```python
from build123d import *

# Parameters (mm, degrees)
SKETCH_1_W          = 29
SKETCH_1_H          = 40
EXTRUDE_1_DEPTH     = 2
SKETCH_2_W          = 2
SKETCH_2_H          = 5
EXTRUDE_2_DEPTH     = 3.5
SKETCH_3_W          = 8.3
SKETCH_3_H          = 3.2
CUT_EXTRUDE_1_DEPTH = 50.71166865
SKETCH_4_R          = 1.9
CUT_EXTRUDE_2_DEPTH = 50.71166865
SKETCH_5_W          = 10.7
SKETCH_5_H          = 5.6
SKETCH_5_W_2        = 8.3
SKETCH_5_H_2        = 3.2
EXTRUDE_3_DEPTH     = 2
SKETCH_6_R          = 3.1
SKETCH_6_R_2        = 1.9
EXTRUDE_4_DEPTH     = 1
EXTRUDE_5_DEPTH     = 1.25
FILLET_1_R          = 0.5
FILLET_2_R          = 0.5
CHAMFER_1_SIZE      = 0.2
CHAMFER_2_SIZE      = 0.5
FILLET_3_R          = 1
FILLET_4_R          = 1
SKETCH_9_W          = 29
SKETCH_9_H          = 19
CUT_EXTRUDE_3_DEPTH = 0.6
FILLET_5_R          = 1


with BuildPart() as part:
    # 草图1 → 凸台-拉伸1 (new body)
    with BuildSketch(Plane.XY):
        with Locations((14.5, 20)):
            Rectangle(SKETCH_1_W, SKETCH_1_H)
    extrude(amount=EXTRUDE_1_DEPTH)

    # 草图2 → 凸台-拉伸2 (add)
    with BuildSketch(Plane(origin=(0, 0, 0), x_dir=(-1, 0, 0), z_dir=(0, 0, -1))):
        with Locations((-1, 34.8)):
            Rectangle(SKETCH_2_W, SKETCH_2_H)
        with Locations((-28, 34.8)):
            Rectangle(SKETCH_2_W, SKETCH_2_H)
        with Locations((-1, 5.2)):
            Rectangle(SKETCH_2_W, SKETCH_2_H)
        with Locations((-28, 5.2)):
            Rectangle(SKETCH_2_W, SKETCH_2_H)
    extrude(amount=EXTRUDE_2_DEPTH)

    # 草图3 → 切除-拉伸1 (cut, through all)
    with BuildSketch(Plane.XY.offset(2)):
        with Locations((14.5, 32.9)):
            Rectangle(SKETCH_3_W, SKETCH_3_H)
    extrude(amount=-CUT_EXTRUDE_1_DEPTH, mode=Mode.SUBTRACT)

    # 草图4 → 切除-拉伸2 (cut, through all)
    with BuildSketch(Plane.XY.offset(2)):
        with Locations((14.5, 5.2)):
            Circle(SKETCH_4_R)
        with Locations((6.2, 5.2)):
            Circle(SKETCH_4_R)
        with Locations((22.8, 5.2)):
            Circle(SKETCH_4_R)
    extrude(amount=-CUT_EXTRUDE_2_DEPTH, mode=Mode.SUBTRACT)

    # 草图5 → 凸台-拉伸3 (add)
    with BuildSketch(Plane(origin=(0, 0, 0), x_dir=(-1, 0, 0), z_dir=(0, 0, -1))):
        with Locations((-14.5, 32.9)):
            Rectangle(SKETCH_5_W, SKETCH_5_H)
        with Locations((-14.5, 32.9)):
            Rectangle(SKETCH_5_W_2, SKETCH_5_H_2, mode=Mode.SUBTRACT)
    extrude(amount=EXTRUDE_3_DEPTH)

    # 草图6 → 凸台-拉伸4 (add)
    with BuildSketch(Plane(origin=(0, 0, 0), x_dir=(-1, 0, 0), z_dir=(0, 0, -1))):
        with Locations((-22.8, 5.2)):
            Circle(SKETCH_6_R)
        with Locations(Location((-22.8, 5.2, 0), (0, 0, 180))):
            Circle(SKETCH_6_R_2, mode=Mode.SUBTRACT)
        with Locations((-14.5, 5.2)):
            Circle(SKETCH_6_R)
        with Locations(Location((-14.5, 5.2, 0), (0, 0, 180))):
            Circle(SKETCH_6_R_2, mode=Mode.SUBTRACT)
        with Locations((-6.2, 5.2)):
            Circle(SKETCH_6_R)
        with Locations(Location((-6.2, 5.2, 0), (0, 0, 180))):
            Circle(SKETCH_6_R_2, mode=Mode.SUBTRACT)
    extrude(amount=EXTRUDE_4_DEPTH)

    # 草图10 → 凸台-拉伸5 (add, symmetric)
    with BuildSketch(Plane(origin=(0, 34.8, 0), x_dir=(-1, 0, 0), z_dir=(0, -1, 0))):
        Polygon((-29, 0.8), (-29.8, 0), (-29, -0.8), align=None)
        Polygon((0, -0.8), (0, 0.8), (0.8, 0), align=None)
    extrude_5 = extrude(amount=EXTRUDE_5_DEPTH, both=True)

    # 镜向1: 凸台-拉伸5 across plane
    add(extrude_5.mirror(Plane(origin=(0, 20, 0), x_dir=(0, 0, 1), z_dir=(0, -1, 0))))

    # 圆角1
    fillet_1_edges = [part.edges().sort_by_distance(p)[0] for p in [
        (29, 37.3, -1.75),
        (29, 32.3, -1.75),
        (27, 32.3, -1.75),
        (27, 37.3, -1.75),
        (0, 37.3, -1.75),
        (2, 37.3, -1.75),
        (2, 32.3, -1.75),
        (0, 32.3, -1.75),
        (0, 2.7, -1.75),
        (0, 7.7, -1.75),
        (2, 7.7, -1.75),
        (2, 2.7, -1.75),
        (29, 2.7, -1.75),
        (27, 2.7, -1.75),
        (27, 7.7, -1.75),
        (29, 7.7, -1.75),
    ]]
    fillet(fillet_1_edges, radius=FILLET_1_R)

    # 圆角2
    fillet_2_edges = [part.edges().sort_by_distance(p)[0] for p in [
        (18.65, 34.5, 0),
        (18.65, 31.3, 0),
        (10.35, 31.3, 0),
        (10.35, 34.5, 0),
    ]]
    fillet(fillet_2_edges, radius=FILLET_2_R)

    # 倒角1
    chamfer_1_edges = [part.edges().sort_by_distance(p)[0] for p in [
        (20.9, 5.2, -1),
        (12.6, 5.2, -1),
        (4.3, 5.2, -1),
    ]]
    chamfer(chamfer_1_edges, length=CHAMFER_1_SIZE)

    # 倒角2
    chamfer_2_edges = [part.edges().sort_by_distance(p)[0] for p in [
        (18.65, 32.9, -2),
        (14.5, 31.3, -2),
        (14.5, 34.5, -2),
        (10.35, 32.9, -2),
        (18.503553391, 31.446446609, -2),
        (18.503553391, 34.353553391, -2),
        (10.496446609, 31.446446609, -2),
        (10.496446609, 34.353553391, -2),
    ]]
    chamfer(chamfer_2_edges, length=CHAMFER_2_SIZE)

    # 圆角3
    fillet_3_edges = [part.edges().sort_by_distance(p)[0] for p in [
        (0, 40, 1),
        (29, 40, 1),
        (29, 0, 1),
        (0, 0, 1),
    ]]
    fillet(fillet_3_edges, radius=FILLET_3_R)

    # 圆角4
    fillet_4_edges = [part.edges().sort_by_distance(p)[0] for p in [
        (19.85, 30.1, -1),
        (9.15, 30.1, -1),
        (9.15, 35.7, -1),
        (19.85, 35.7, -1),
    ]]
    fillet(fillet_4_edges, radius=FILLET_4_R)

    # 草图9 → 切除-拉伸3 (cut)
    with BuildSketch(Plane(origin=(0, 0, 0), x_dir=(-1, 0, 0), z_dir=(0, 0, -1))):
        with Locations((-14.5, 20)):
            Rectangle(SKETCH_9_W, SKETCH_9_H)
    extrude(amount=-CUT_EXTRUDE_3_DEPTH, mode=Mode.SUBTRACT)

    # 圆角5
    fillet_5_edges = [part.edges().sort_by_distance(p)[0] for p in [
        (29, 10.5, 0.3),
        (29, 29.5, 0.3),
        (0, 29.5, 0.3),
        (0, 10.5, 0.3),
    ]]
    fillet(fillet_5_edges, radius=FILLET_5_R)


solid = part.part
```
Part model, mm, in its own coordinate system. A direction names the side the tool comes from. Round coordinates to 2 decimals unless told otherwise and drop trailing zeros. Order: outer loops, then holes, each group sorted by start corner. A loop starts at its lowest first (then second) coordinate and runs counter-clockwise, first axis right, second up. Notation, with made-up numbers: M 9,-22.5 L 20,-22.5 A22 cw 20,3.5 Z; hole C 17,47 d2. An arc over 180 degrees is marked long. Answer in a Markdown table with one row per item. Add a question column.
Q1. Cut at B-B on x = 6.2. Give the cut face in (y, z), and give its area (3 significant figures).
Q2. Cut at D-D on z = 1.3. Give the cut face in (x, y), and give its area (3 significant figures).
Q3. Mould opens along Y. For faces 5 (the face through (10.35, 31.31, -1.7)), 6 (the face through (-0.3, 36.05, 0)), 7 (the face through (22, 3, -1)) say: +Y half, -Y half, draft (parallel to the pull), parting line (faces both ways), or undercut.
Q4. Pin check, flat tips, straight feed: pin 1 (1 mm diameter, centred on y = 5.5, z = -2, fed in from -X); pin 2 (0.6 mm diameter, centred on x = 29.5, z = 0, fed in from +Y); pin 3 (0.8 mm diameter, centred on x = 28, z = -1, fed in from -Y); pin 4 (2.5 mm diameter, centred on x = 6.2, y = 5.2, fed in from -Z). Stop position of each tip, or through.
Q5. Cut at C-C on z = -2.7. Give the number of separate pieces and of enclosed holes in the cut face, and give its area (3 significant figures).
Q6. 3-axis set-ups, long thin cutter, end or side, ignore diameter. For faces 1 (the face through (29.3, 3.95, 0)), 2 (the face through (15, 35.7, -1)), 3 (the face through (28, 37.3, -2)), 4 (the face through (10.36, 34.5, -1.7)): which of +Z, -Z, +X, -X, +Y, -Y reach the whole face in a straight line?
Q7. Cut at A-A on x = 14.5. Give the cut face in (y, z).
Q8. Wall check: L1, parallel to Y at x = 14.5, z = -0.4; L2, parallel to Y at x = 1.5, z = -3.05; L3, parallel to X at y = 6.5, z = -2.2. Give the ranges that are in metal, low to high. Write a range as from..to.
Established:
| question | item | result |
|---|---|---|
| 1 | outline | M 0,0 L 2.1,0 L 2.1,-1 L 3.1,-1 L 3.3,-0.8 L 3.3,2 L 0,2 Z; M 7.1,-0.8 L 7.3,-1 L 8.3,-1 L 8.3,0 L 10.5,0 L 10.5,0.6 L 29.5,0.6 L 29.5,0 L 40,0 L 40,2 L 7.1,2 Z |
| 1 | area | 63.4 mm2 |
| 2 | outline | M 0,1 A1 ccw 1,0 L 28,0 A1 ccw 29,1 L 29,39 A1 ccw 28,40 L 1,40 A1 ccw 0,39 Z; hole C 6.2,5.2 d3.8; hole M 10.35,31.8 A0.5 ccw 10.85,31.3 L 18.15,31.3 A0.5 ccw 18.65,31.8 L 18.65,34 A0.5 ccw 18.15,34.5 L 10.85,34.5 A0.5 ccw 10.35,34 Z; hole C 14.5,5.2 d3.8; hole C 22.8,5.2 d3.8 |
| 2 | area | 1,100 mm2 |
| 3 | face 5 | undercut |
| 3 | face 6 | +Y half |
| 3 | face 7 | draft |
| 4 | pin 1 | stops at x = 0 |
| 4 | pin 2 | stops at y = 36.05 |
| 4 | pin 3 | stops at y = 2.7 |
| 4 | pin 4 | passes through |
| 5 | separate pieces | 4 |
| 5 | enclosed holes | 0 |
| 5 | area | 39.1 mm2 |
| 6 | face 1 | +Z, -Z, +X, -Y |
| 6 | face 2 | -Z, +Y |
| 6 | face 3 | -Z, +X, -X, +Y |
| 6 | face 4 | -Z |
| 7 | outline | M 0,0 L 2.1,0 L 2.1,-1 L 3.1,-1 L 3.3,-0.8 L 3.3,2 L 0,2 Z; M 7.1,-0.8 L 7.3,-1 L 8.3,-1 L 8.3,0 L 10.5,0 L 10.5,0.6 L 29.5,0.6 L 29.5,0 L 30.1,0 L 30.1,-2 L 30.8,-2 L 31.3,-1.5 L 31.3,2 L 7.1,2 Z; M 34.5,-1.5 L 35,-2 L 35.7,-2 L 35.7,0 L 40,0 L 40,2 L 34.5,2 Z |
| 8 | L1 | y = 2.1..3.3, 7.1..8.3, 30.1..31.3, 34.5..35.7 |
| 8 | L2 | y = 2.7..7.7, 32.3..37.3 |
| 8 | L3 | x = 0..2, 27..29 |
